Autodesk Inventor part; units mm, degrees
ref_plane "Work Plane1" through (0, 76.2, 0) normal (0, 1, 0) x (-1, 0, 0)
ref_plane "YZ Plane" through (0, 0, 0) normal (1, 0, 0) x (0, 1, 0)
ref_plane "XY Plane" through (0, 0, 0) normal (0, 0, 1) x (1, 0, 0)
sketch "Sketch1" plane through (0, 0, 0) normal (0, 1, 0) x (-1, 0, 0)
  circle A0 centre (0, 0) radius 76.2 construction
  line L0 (0, 0) -> (0, 76.2) construction
  line L1 (0, 0) -> (65.9911, -38.1) construction
  line L2 (0, 0) -> (-65.9911, -38.1) construction
  dimension "d0" = 152.4
  dimension "d1" = 120
  dimension "d2" = 120
sketch "Sketch2" plane through (0, 0, 0) normal (1, 0, 0) x (0, 1, 0)
  line L0 (0, 0) -> (76.2, 0) construction
  dimension "d3" = 76.2
ref_plane "Work Plane1" through (0, 76.2, 0) normal (0, 1, 0) x (-1, 0, 0)
sketch "Sketch3" plane through (0, 76.2, 0) normal (0, 1, 0) x (-1, 0, 0)
  circle A0 centre (0, 0) radius 12.7
  dimension "d5" = 25.4
sketch3d "3D Sketch1"
  line L0 (0, 76.2, 0) -> (0, 0, 76.2)
sweep "Sweep2" add profiles "Sketch3" path "3D Sketch1"
sketch "Sketch4" plane through (0, 76.2, 0) normal (0, 1, 0) x (-1, 0, 0)
  circle A0 centre (0, 0) radius 12.7
sketch3d "3D Sketch2"
  line L0 (0, 76.2, 0) -> (65.9911, 0, -38.1)
sweep "Sweep3" add profiles "Sketch4" path "3D Sketch2"
sketch "Sketch5" plane through (0, 76.2, 0) normal (0, 1, 0) x (-1, 0, 0)
  circle A0 centre (0, 0) radius 12.7
sketch3d "3D Sketch3"
  line L0 (0, 76.2, 0) -> (-65.9911, 0, -38.1)
sweep "Sweep4" add profiles "Sketch5" path "3D Sketch3"
properties part number "CameraTripodBase"
Design review of the part built by this model. Coordinates are the model's own, in mm. Round coordinates to 2 decimals unless told otherwise and drop trailing zeros.
1) For L1, parallel to X at y = 34, z = -13; L2, parallel to X at y = 48, z = -7; L3, parallel to Y at x = -36, z = -17, list the stretches that pass through material, from the lowest coordinate up.
The answers:
L1: x = -46.33 to -26.76, 26.76 to 46.33
L2: x = -34.95 to -13.89, 13.89 to 34.95
L3: y = 24.25 to 48.79
2) Clearance check with flat-ended pins moving along their axes: pin 1 Ø10 at (y, z) = (55, 18) entering from -X; pin 2 Ø1 at (y, z) = (12.5, 61) entering from -X; pin 3 Ø1.5 at (y, z) = (39.5, 47) entering from -X; pin 4 Ø1 at (x, z) = (14, 35.5) entering from +Y. State where each tip first meets the part, or that it passes through.
The answers:
pin 1: stops at x = -12.7
pin 2: stops at x = -12.54
pin 3: stops at x = -8.71
pin 4: passes through
3) Consider section A-A (y = 19.5). Count the separate pieces of the cut face and the enclosed holes in it, plus the area to 3 significant figures.
The answers:
separate pieces: 3
enclosed holes: 0
area: 1,520 mm2
